Here's how the part is built. I have some questions about the finished solid (model axes, mm). Face numbers are marked on the shaded views. Coordinates: 2 decimals unless noted, no trailing zeros. Write each loop counter-clockwise with the first axis right and the second up, starting at its lowest first coordinate (ties: lowest second). Pieces come first, ordered by that corner, then holes.
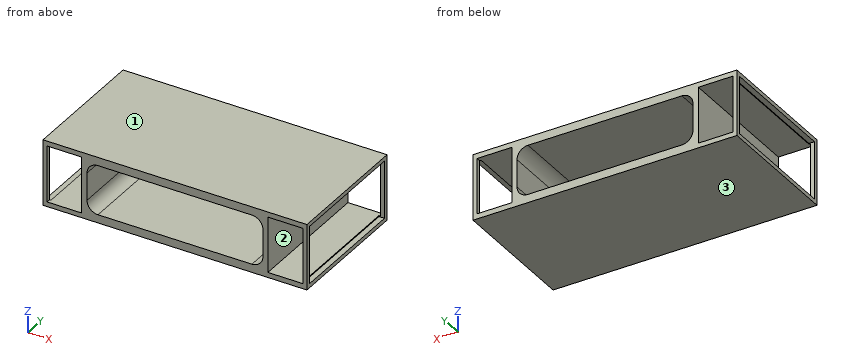
```python
from build123d import *

# Parameters (mm, degrees)
F0_W     = 1219.2
F0_H     = 609.6
F1_DEPTH = 152.4
F3_DEPTH = 1219.2
F4_W     = 161.274815
F4_H     = 257.426903
F4_W_2   = 159.263874
F4_H_2   = 260.308549
F5_DEPTH = 1219.2
F6_W     = 571.5
F6_H     = 266.7
F7_DEPTH = 25.4
F8_W     = 571.5
F8_H     = 266.7
F9_DEPTH = 25.4


with BuildPart() as f1:
    # F0 (on Top) → F1 (new body, symmetric)
    with BuildSketch(Plane.XY):
        Rectangle(F0_W, F0_H)
    extrude(amount=F1_DEPTH, both=True)

    # F2 (on face) → F3 (cut)
    with BuildSketch(Plane.XZ.offset(304.8)):
        with BuildLine():
            Line((-355.6, -114.3), (355.6, -114.3))
            ThreePointArc((355.6, -114.3), (391.521024, -99.421024), (406.4, -63.5))
            Line((406.4, -63.5), (406.4, 63.5))
            ThreePointArc((406.4, 63.5), (391.521024, 99.421024), (355.6, 114.3))
            Line((355.6, 114.3), (-355.6, 114.3))
            ThreePointArc((-355.6, 114.3), (-391.521024, 99.421024), (-406.4, 63.5))
            Line((-406.4, 63.5), (-406.4, -63.5))
            ThreePointArc((-406.4, -63.5), (-391.521024, -99.421024), (-355.6, -114.3))
        make_face()
    extrude(amount=-F3_DEPTH, mode=Mode.SUBTRACT)

    # F4 (on face) → F5 (cut)
    with BuildSketch(Plane.XZ.offset(304.8)):
        with Locations((509.912592, 0.053682)):
            Rectangle(F4_W, F4_H)
        with Locations((-510.918063, -0.480272)):
            Rectangle(F4_W_2, F4_H_2)
    extrude(amount=-F5_DEPTH, mode=Mode.SUBTRACT)

    # F6 (on face) → F7 (cut)
    with BuildSketch(Plane.YZ.offset(609.6)):
        Rectangle(F6_W, F6_H)
    extrude(amount=-F7_DEPTH, mode=Mode.SUBTRACT)

    # F8 (on face) → F9 (cut)
    with BuildSketch(Plane(origin=(-609.6, 0, 0), x_dir=(0, -1, 0), z_dir=(-1, 0, 0))):
        Rectangle(F8_W, F8_H)
    extrude(amount=-F9_DEPTH, mode=Mode.SUBTRACT)


solid = f1.part
```
1) Imagine slicing it at B-B on z = 24.5. Please give me the cut outline in (x, y).
Values follow:
outline: (-609.6, -304.8) - (-590.55, -304.8) - (-590.55, -285.75) - (-609.6, -285.75) - close; (-609.6, 285.75) - (-590.55, 285.75) - (-590.55, 304.8) - (-609.6, 304.8) - close; (-431.29, -304.8) - (-406.4, -304.8) - (-406.4, 304.8) - (-431.29, 304.8) - close; (406.4, -304.8) - (429.28, -304.8) - (429.28, 304.8) - (406.4, 304.8) - close; (590.55, -304.8) - (609.6, -304.8) - (609.6, -285.75) - (590.55, -285.75) - close; (590.55, 285.75) - (609.6, 285.75) - (609.6, 304.8) - (590.55, 304.8) - close
2) Imagine slicing it at A-A on x = 448. Please give me the cut outline in (y, z).
Values follow:
outline: (-304.8, -152.4) - (304.8, -152.4) - (304.8, -128.66) - (-304.8, -128.66) - close; (-304.8, 128.77) - (304.8, 128.77) - (304.8, 152.4) - (-304.8, 152.4) - close
3) Will these pins go through, and if not, where does the flat tip stop? pin 1 (1.4 mm diameter, centred on y = 91, z = -131.5, fed in from -X); pin 2 (2.5 mm diameter, centred on y = 26, z = 131, fed in from +X); pin 3 (6 mm diameter, centred on y = 114, z = 31, fed in from -X).
Values follow:
pin 1: stops at x = -584.2
pin 2: stops at x = 584.2
pin 3: stops at x = -431.29
4) I need wall thicknesses on probe 1 along Z at (x, y) = (-433, -158); probe 2 along Z at (x, y) = (-298, -127); probe 3 along X at (y, z) = (214, 45.5). Which ranges of each line are inside material? Lowest first, please.
Values follow:
probe 1: z = -152.4 to -130.63, 129.67 to 152.4
probe 2: z = -152.4 to -114.3, 114.3 to 152.4
probe 3: x = -431.29 to -406.4, 406.4 to 429.28
5) We'd pull the mould along Z, two halves only. Please class the marked faces 1, 2 and 3: pulls with the +Z half, pulls with the -Z half, needs draft (parallel to the pull), parting line crosses it, or undercut.
Values follow:
face 1: pulls with the +Z half
face 2: undercut
face 3: pulls with the -Z half
6) Imagine slicing it at D-D on x = -332. Please give me the cut outline in (y, z), then the cut area to 3 significant figures.
Values follow:
outline: (-304.8, -152.4) - (304.8, -152.4) - (304.8, -114.3) - (-304.8, -114.3) - close; (-304.8, 114.3) - (304.8, 114.3) - (304.8, 152.4) - (-304.8, 152.4) - close
area: 46,500 mm2
7) Imagine slicing it at C-C on y = -33. Please give me the cut outline in (x, z).
Values follow:
outline: (-609.6, -152.4) - (609.6, -152.4) - (609.6, -133.35) - (584.2, -133.35) - (584.2, -128.66) - (429.28, -128.66) - (429.28, 128.77) - (584.2, 128.77) - (584.2, 133.35) - (609.6, 133.35) - (609.6, 152.4) - (-609.6, 152.4) - (-609.6, 133.35) - (-584.2, 133.35) - (-584.2, 129.67) - (-431.29, 129.67) - (-431.29, -130.63) - (-584.2, -130.63) - (-584.2, -133.35) - (-609.6, -133.35) - close; hole (-406.4, -63.5) arc R50.8 ccw to (-355.6, -114.3) - (355.6, -114.3) arc R50.8 ccw to (406.4, -63.5) - (406.4, 63.5) arc R50.8 ccw to (355.6, 114.3) - (-355.6, 114.3) arc R50.8 ccw to (-406.4, 63.5) - close
